Geometry check sheet. Reference: the model listing, model coordinates, mm. A direction names the side the tool comes from. Round coordinates to 2 decimals unless told otherwise and drop trailing zeros. Loops run counter-clockwise (first coordinate to the right, second up) from the corner with the lowest first, then second, coordinate; pieces in that order, holes last. Notation, with made-up numbers: (6.25, 63) - (11.25, 63) arc R4 ccw to (11.25, 68) - close; hole circle Ø4 at (1.25, -31). An arc over 180 degrees is marked (long way). Answer as CSV lines item,"result". Start each with the question number.
1) Cross-section at A-A on y = 5.75. Record the boundary of the cut face in (x, z).
2) Cross-section at C-C on x = 2.25. Record the boundary of the cut face in (y, z), and give its area (3 significant figures).
3) Cross-section at B-B on x = 8.75. Record the boundary of the cut face in (y, z).
4) Access from +Z, -Z, +X, -X, +Y, -Y to the whole of each face (thin tool, end or side, straight path). Record for faces 1 (the flat face through (5.5, -9.4, 7.874)), 2 (the cylindrical face through (-10.646, -0.684, 0.11)).
5) Draft check along X on faces 3 (the flat face through (5.5, -9.4, -7.874)), 4 (the cylindrical face through (-0.081, -15.784, 0.11)), 5 (the cylindrical face through (10.66, -0.38, 0.11)). Enter one of: released by +X, released by -X, zero draft, split by the parting line, or undercut.
6) Depth check by flat-ended pin: P1, Ø2, axis at x = 5, z = 2, coming from the -Y side; P2, Ø1, axis at x = 4, z = -2, coming from the +Y side; P3, Ø5, axis at y = -5, z = 3, coming from the +X side. Enter the tip coordinate at first touch or a pass-through.
7) Thickness scan on line 1 along Y through (x, z) = (8.5, -2.5); line 2 along X through (y, z) = (-6.5, -7); line 3 along X through (y, z) = (5, -1.75). Record the ranges inside material, lowest first.
from build123d import *

# Parameters (mm, degrees)
F1_DEPTH = 7.874
F2_R     = 5.08


# Not quite as in the source:
# - a feature names something its author has since deleted; it is built from what else it names


with BuildPart() as f1:
    # F0 (on Top) → F1 (new body, symmetric)
    with BuildSketch(Plane.XY):
        with BuildLine():
            ThreePointArc((-3.175, -10.1845765253), (-10.541007581, -1.6411530025), (-6.1209836066, 8.7372640848))
            ThreePointArc((-6.1209836066, 8.7372640848), (-5.8873871353, 10.063893343), (-7.2140163934, 10.2974898143))
            ThreePointArc((-7.2140163934, 10.2974898143), (-12.5113475889, -1.2435877575), (-5.0458178338, -11.5160779516))
            ThreePointArc((-5.0458178338, -11.5160779516), (0, -15.7845920127), (5.0458178338, -11.5160779516))
            ThreePointArc((5.0458178338, -11.5160779516), (12.5113475889, -1.2435877575), (7.2140163934, 10.2974898143))
            ThreePointArc((7.2140163934, 10.2974898143), (5.8873871353, 10.063893343), (6.1209836066, 8.7372640848))
            ThreePointArc((6.1209836066, 8.7372640848), (10.541007581, -1.6411530025), (3.175, -10.1845765253))
            ThreePointArc((3.175, -10.1845765253), (0, -13.8795920127), (-3.175, -10.1845765253))
        make_face()
    extrude(amount=F1_DEPTH, both=True)

    # F2
    f2_edges = [f1.edges().sort_by_distance(p)[0] for p in [
        (-5.045818, -11.516078, 0),
        (-3.175, -10.184577, 0),
        (3.175, -10.184577, 0),
        (5.045818, -11.516078, 0),
    ]]
    fillet(f2_edges, radius=F2_R)


solid = f1.part
Answer block:
1,outline,"(-11.18, -7.87) - (-8.99, -7.87) - (-8.99, 7.87) - (-11.18, 7.87) - close; (8.99, -7.87) - (11.18, -7.87) - (11.18, 7.87) - (8.99, 7.87) - close"
2,outline,"(-15.26, -7.87) - (-12.96, -7.87) - (-12.96, 7.87) - (-15.26, 7.87) - close"
2,area,"36.3 mm^2"
3,outline,"(-9.03, -7.87) - (-6.1, -7.87) - (-6.1, 7.87) - (-9.03, 7.87) - close; (6.1, -7.87) - (9.03, -7.87) - (9.03, 7.87) - (6.1, 7.87) - close"
4,face 1,"+Z, +X, -X, +Y, -Y"
4,face 2,"+Z, -Z"
5,face 3,"zero draft"
5,face 4,"split by the parting line"
5,face 5,"undercut"
6,P1,"stops at y = -13.86"
6,P2,"stops at y = -9.79"
6,P3,"stops at x = 12.32"
7,line 1,"y = -9.26 to -6.45, 6.45 to 9.26"
7,line 2,"x = -10.76 to -8.46, 8.46 to 10.76"
7,line 3,"x = -11.54 to -9.42, 9.42 to 11.54"
